```python
from build123d import *

# Parameters (mm, degrees)
F0_W         = 144
F0_H         = 22
F1_DEPTH     = 2
F3_DEPTH     = 25
F5_DEPTH     = 160
F6_T1_DEPTH  = 18
F6_T3_DEPTH  = 140
F6_T5_DEPTH  = 30
F6_T7_DEPTH  = 39.6649624979
F6_T9_DEPTH  = 8
F6_T11_DEPTH = 154
F6_S15_W     = 2
F6_S15_H     = 2
F6_T16_DEPTH = 2
F6_S21_W     = 2
F6_S21_H     = 2
F6_T22_DEPTH = 2
F6_S27_W     = 2
F6_S27_H     = 2
F6_T28_DEPTH = 2
F6_S33_W     = 2
F6_S33_H     = 2
F6_T34_DEPTH = 2


# Not quite as in the source:
# - a fillet or chamfer that OpenCascade refuses, or shapes differently, is made with other operations: its cross-section is extruded or revolved along the edge and cut away or added


with BuildPart() as f1:
    # F0 (on Top) → F1 (new body)
    with BuildSketch(Plane.XY):
        Rectangle(F0_W, F0_H)
    extrude(amount=F1_DEPTH)

    # F2 (on face) → F3 (join)
    with BuildSketch(Plane.XY.offset(2)):
        Polygon((-70.000000298, -11), (-70.000000298, 9.000000298), (70.000000298, 9.000000298), (70.000000298, -11), (72, -11), (72, 11), (-72, 11), (-72, -11), align=None)
    extrude(amount=F3_DEPTH)

    # F4 (on face) → F5 (cut)
    with BuildSketch(Plane(origin=(-72, 0, 0), x_dir=(0, -1, 0), z_dir=(-1, 0, 0))):
        Polygon((11, 27), (-8.9, 27), (11, 5), align=None)
    extrude(amount=-F5_DEPTH, mode=Mode.SUBTRACT)

    # F6: fillet of radius 2 on 11 edges, made by hand

    # F6_s2 → F6_t1 (cut)
    with BuildSketch(Plane.XZ.offset(-9)):
        with BuildLine():
            ThreePointArc((72, 2), (71.4142135624, 0.5857864376), (70, 0))
            Line((70, 0), (72, 0))
            Line((72, 0), (72, 2))
        make_face()
        with BuildLine():
            ThreePointArc((-70, 0), (-71.4142135624, 0.5857864376), (-72, 2))
            Line((-72, 2), (-72, 0))
            Line((-72, 0), (-70, 0))
        make_face()
    extrude(amount=F6_T1_DEPTH, mode=Mode.SUBTRACT)

    # F6_s4 → F6_t3 (cut)
    with BuildSketch(Plane.YZ.offset(-70)):
        with BuildLine():
            ThreePointArc((9, 0), (10.4142135624, 0.5857864376), (11, 2))
            Line((11, 2), (11, 0))
            Line((11, 0), (9, 0))
        make_face()
        with BuildLine():
            ThreePointArc((-11, 2), (-10.4142135624, 0.5857864376), (-9, 0))
            Line((-9, 0), (-11, 0))
            Line((-11, 0), (-11, 2))
        make_face()
    extrude(amount=F6_T3_DEPTH, mode=Mode.SUBTRACT)

    # F6_s6 → F6_t5 (cut)
    with BuildSketch(Plane.XY.offset(2)):
        with BuildLine():
            ThreePointArc((-70, 11), (-71.4142135624, 10.4142135624), (-72, 9))
            Line((-72, 9), (-72, 11))
            Line((-72, 11), (-70, 11))
        make_face()
        with BuildLine():
            ThreePointArc((72, 9), (71.4142135624, 10.4142135624), (70, 11))
            Line((70, 11), (72, 11))
            Line((72, 11), (72, 9))
        make_face()
    extrude(amount=F6_T5_DEPTH, mode=Mode.SUBTRACT)

    # F6_s8 → F6_t7 (cut)
    with BuildSketch(Plane(origin=(0, 20.7915282423, 22.9856091121), x_dir=(1, 0, 0), z_dir=(0, -0.6708250517, -0.741615635))):
        with BuildLine():
            ThreePointArc((72, 9.5118972432), (71.4142135624, 10.9261108056), (70, 11.5118972432))
            Line((70, 11.5118972432), (72, 11.5118972432))
            Line((72, 11.5118972432), (72, 9.5118972432))
        make_face()
        with BuildLine():
            ThreePointArc((-72, 9.5118972432), (-71.4142135624, 10.9261108056), (-70, 11.5118972432))
            Line((-70, 11.5118972432), (-72, 11.5118972432))
            Line((-72, 11.5118972432), (-72, 9.5118972432))
        make_face()
    extrude(amount=F6_T7_DEPTH, mode=Mode.SUBTRACT)

    # F6_s10 → F6_t9 (cut)
    with BuildSketch(Plane.XY.offset(2)):
        with BuildLine():
            ThreePointArc((-70, -11), (-71.4142135624, -10.4142135624), (-72, -9))
            Line((-72, -9), (-72, -11))
            Line((-72, -11), (-70, -11))
        make_face()
        with BuildLine():
            ThreePointArc((72, -9), (71.4142135624, -10.4142135624), (70, -11))
            Line((70, -11), (72, -11))
            Line((72, -11), (72, -9))
        make_face()
    extrude(amount=F6_T9_DEPTH, mode=Mode.SUBTRACT)

    # F6_s12 → F6_t11 (cut)
    with BuildSketch(Plane.YZ.offset(-77)):
        with BuildLine():
            ThreePointArc((11, 25), (10.4142135624, 26.4142135624), (9, 27))
            Line((9, 27), (11, 27))
            Line((11, 27), (11, 25))
        make_face()
    extrude(amount=F6_T11_DEPTH, mode=Mode.SUBTRACT)


with BuildPart() as f6_tool14:
    # F6_s15 → F6_t16 (new body)
    with BuildSketch(Plane.YZ.offset(70)):
        with Locations((-10, 1)):
            Rectangle(F6_S15_W, F6_S15_H)
    extrude(amount=F6_T16_DEPTH)

    # F6_s17 → F6_t18 (revolve, cut)
    with BuildSketch(Plane(origin=(70, -9, 2), x_dir=(0, 0.7071067812, 0.7071067812), z_dir=(0, 0.7071067812, -0.7071067812))):
        with BuildLine():
            ThreePointArc((0, -2), (2, 0), (0, 2))
            Line((0, 2), (0, -2))
        make_face()
    revolve(axis=Axis((70, -9, 2), (1, 0, 0)), mode=Mode.SUBTRACT)


with BuildPart() as f1_1:
    add(f1.part)

    # F6_t13: cut F6_tool14
    add(f6_tool14.part, mode=Mode.SUBTRACT)


with BuildPart() as f6_tool20:
    # F6_s21 → F6_t22 (new body)
    with BuildSketch(Plane.YZ.offset(70)):
        with Locations((10, 1)):
            Rectangle(F6_S21_W, F6_S21_H)
    extrude(amount=F6_T22_DEPTH)

    # F6_s23 → F6_t24 (revolve, cut)
    with BuildSketch(Plane(origin=(70, 9, 2), x_dir=(0, -0.7071067812, 0.7071067812), z_dir=(0, 0.7071067812, 0.7071067812))):
        with BuildLine():
            ThreePointArc((0, -2), (2, 0), (0, 2))
            Line((0, 2), (0, -2))
        make_face()
    revolve(axis=Axis((70, 9, 2), (1, 0, 0)), mode=Mode.SUBTRACT)


with BuildPart() as f1_2:
    add(f1_1.part)

    # F6_t19: cut F6_tool20
    add(f6_tool20.part, mode=Mode.SUBTRACT)


with BuildPart() as f6_tool26:
    # F6_s27 → F6_t28 (new body)
    with BuildSketch(Plane.XY.offset(2)):
        with Locations((-71, 10)):
            Rectangle(F6_S27_W, F6_S27_H)
    extrude(amount=-F6_T28_DEPTH)

    # F6_s29 → F6_t30 (revolve, cut)
    with BuildSketch(Plane(origin=(-70, 9, 2), x_dir=(0.7071067812, -0.7071067812, 0), z_dir=(0.7071067812, 0.7071067812, 0))):
        with BuildLine():
            ThreePointArc((0, -2), (2, 0), (0, 2))
            Line((0, 2), (0, -2))
        make_face()
    revolve(axis=Axis((-70, 9, 2), (0, 0, -1)), mode=Mode.SUBTRACT)


with BuildPart() as f1_3:
    add(f1_2.part)

    # F6_t25: cut F6_tool26
    add(f6_tool26.part, mode=Mode.SUBTRACT)


with BuildPart() as f6_tool32:
    # F6_s33 → F6_t34 (new body)
    with BuildSketch(Plane.XZ.offset(9)):
        with Locations((-71, 1)):
            Rectangle(F6_S33_W, F6_S33_H)
    extrude(amount=F6_T34_DEPTH)

    # F6_s35 → F6_t36 (revolve, cut)
    with BuildSketch(Plane(origin=(-70, -9, 2), x_dir=(0.7071067812, 0, 0.7071067812), z_dir=(0.7071067812, 0, -0.7071067812))):
        with BuildLine():
            ThreePointArc((0, -2), (2, 0), (0, 2))
            Line((0, 2), (0, -2))
        make_face()
    revolve(axis=Axis((-70, -9, 2), (0, -1, 0)), mode=Mode.SUBTRACT)


with BuildPart() as f1_4:
    add(f1_3.part)

    # F6_t31: cut F6_tool32
    add(f6_tool32.part, mode=Mode.SUBTRACT)


solid = f1_4.part
```
CAD build for the part. Positions are in the model's coordinates, mm. A direction names the side the tool comes from. Coordinates: 2 decimals unless noted, no trailing zeros. Order: outer loops, then holes, each group sorted by start corner. A loop starts at its lowest first (then second) coordinate and runs counter-clockwise, first axis right, second up. Notation, with made-up numbers: (-34, -15.5) - (-29, -15.5) arc R17 cw to (-29, -0.5) - close; hole circle Ø6 at (50, 19). An arc over 180 degrees is marked (long way). Use a Markdown table: item, result. Add a question column.
(1) Pull direction X, two halves, no side cores. Call faces 3 (the face through (71.43, -0.28, 15.95)), 4 (the face through (-1, 0, 0)), 5 (the face through (70, 1, 12)): +X half, -X half, draft (parallel to the pull), parting line (faces both ways), or undercut.
(2) Flat gauge pins, fed straight in: pin 1 (1 mm diameter, centred on x = -8, y = 1, fed in from +Z); pin 2 (12.5 mm diameter, centred on x = 22, z = 19, fed in from -Y). Where does each tip first touch, or does it go through?
(3) Which spindle directions (+Z, -Z, +X, -X, +Y, -Y) get a long thin tool onto all of the face, cutting with end or side? Do faces 1 (the face through (-71.43, -0.28, 15.95)), 2 (the face through (-70, 1, 12)). Say none if no direction does.
(4) Drill centre lines: line 1 along X through (y, z) = (2.25, 12.5); line 2 along Y through (x, z) = (-53, 17.25); line 3 along Z through (x, y) = (-62, -5.5). Where is each one in solid material? Low to high. Write a range as [from, to].
(5) Saw through at A-A (x = -5.5). Give the cut face in (y, z).
Solved:
| question | item | result |
|---|---|---|
| 1 | face 3 | +X half |
| 1 | face 4 | draft |
| 1 | face 5 | undercut |
| 2 | pin 1 | stops at z = 2 |
| 2 | pin 2 | stops at y = 9 |
| 3 | face 1 | +Z, -X, -Y |
| 3 | face 2 | +Z, -Y |
| 4 | line 1 | x = [-72, -70], [70, 72] |
| 4 | line 2 | y = [9, 11] |
| 4 | line 3 | z = [0, 2] |
| 5 | outline | (-11, 2) arc R2 ccw to (-9, 0) - (9, 0) arc R2 ccw to (11, 2) - (11, 25) arc R2 ccw to (9, 27) - (9, 2) - close |
